The listing builds one solid part. Answer for the finished solid, in the listing's coordinates (mm). A direction names the side the tool comes from. Coordinates: 2 decimals unless noted, no trailing zeros. Write each loop counter-clockwise with the first axis right and the second up, starting at its lowest first coordinate (ties: lowest second). Pieces come first, ordered by that corner, then holes.
(1) For a pull along Z with two mould halves and no side action, classify faces 1 (the cylindrical face through (20.147, 0.986, -61.81)), 2 (the flat face through (-15.21, 0.99, 15.74)), 3 (the cylindrical face through (26.89, 0.99, 52.55)) as +Z half, -Z half, draft (parallel to the pull), parting line (faces both ways), or undercut.
(2) The part is cut by section B-B on y = 1.35. Give the number of separate pieces and of enclosed holes in the cut face, plus the area to 3 significant figures.
(3) Straight lines are drawn through the part: line 1 (X direction, y = 0.9, z = -4.5); line 2 (Z direction, x = 11, y = 0.45) (3 decimals); line 3 (Z direction, x = 3.5, y = 1.3). For each, find the intervals that lie inside material, in ascending order.
(4) The part is cut by section C-C on z = -32. Determine the outline of the cut face in (x, y), plus the area to 3 significant figures.
(5) The part is cut by section A-A on z = 9. Determine the outline of the cut face in (x, y).
(6) Which of the six approach directions +Z, -Z, +X, -X, +Y, -Y give full straight-line access (tool end or side, diameter ignored) to faces 4 (the cylindrical face through (-13.676, 0.986, 38.995)), 5 (the flat face through (35.57, 0.99, -25.22))?
(7) Given P1, Ø4, axis at x = -7.79, z = -4.5, coming from the -Y side, flat-ended and moving along its own axis, determine where the tip first touches the part or whether it passes through.
from build123d import *

# Parameters (mm, degrees)
SKETCH_1_R          = 1.65
SKETCH_1_R_2        = 5.5
EXTRUDE_1_DEPTH     = 2
SKETCH_2_R          = 1.65
CUT_EXTRUDE_1_DEPTH = 86.784644099
FILLET_1_R          = 2


with BuildPart() as part:
    # Эскиз1 → Бобышка-Вытянуть1 (new body)
    with BuildSketch(Plane(origin=(0, 0, 0), x_dir=(1, 0, 0), z_dir=(0, 1, 0))):
        with BuildLine():
            Line((22.63058135, 57.022094922), (48.869113703, -7.475462073))
            ThreePointArc((48.869113703, -7.475462073), (51.017863934, -22.940417651), (45.538728547, -37.5609872))
            ThreePointArc((45.538728547, -37.5609872), (26.585605536, -52.704925153), (3.142096023, -58.946847156))
            ThreePointArc((3.142096023, -58.946847156), (-19.13330087, -49.051718647), (-20.218209383, -24.701567755))
            Line((-20.218209383, -24.701567755), (-10.065450366, -6.533506633))
            ThreePointArc((-10.065450366, -6.533506633), (-6.891228037, 9.824000007), (9.569842381, 7.24003569))
            ThreePointArc((9.569842381, 7.24003569), (16.257964509, 34.227304723), (6.907279065, 60.411428714))
            ThreePointArc((6.907279065, 60.411428714), (9.487905153, 68.030832797), (17.329317504, 66.234391334))
            ThreePointArc((17.329317504, 66.234391334), (20.184340604, 61.745861093), (22.63058135, 57.022094922))
        make_face()
        with Locations(Location((9.550649772, -54.164426416, 0), (0, 0, 270))):
            Circle(SKETCH_1_R, mode=Mode.SUBTRACT)
        with Locations(Location((31.546703999, -45.053362436, 0), (0, 0, 90))):
            Circle(SKETCH_1_R, mode=Mode.SUBTRACT)
        with Locations(Location((0, 0, 0), (0, 0, 270))):
            Circle(SKETCH_1_R_2, mode=Mode.SUBTRACT)
        with Locations(Location((0, -9, 0), (0, 0, 270))):
            Circle(SKETCH_1_R, mode=Mode.SUBTRACT)
        with Locations(Location((-7.794228634, 4.5, 0), (0, 0, 270))):
            Circle(SKETCH_1_R, mode=Mode.SUBTRACT)
        with Locations(Location((7.794228634, 4.5, 0), (0, 0, 270))):
            Circle(SKETCH_1_R, mode=Mode.SUBTRACT)
        with BuildLine():
            Line((-5.357568053, -23.065686545), (20.09827607, -12.521530668))
            ThreePointArc((20.09827607, -12.521530668), (37.096418695, -17.67786086), (35.355339059, -35.355339059))
            ThreePointArc((35.355339059, -35.355339059), (19.134171618, -46.193976626), (0, -50))
            ThreePointArc((0, -50), (-13.730993926, -38.731264508), (-5.357568053, -23.065686545))
        make_face(mode=Mode.SUBTRACT)
    extrude(amount=EXTRUDE_1_DEPTH)

    # Эскиз2 → Вырез-Вытянуть1 (cut, through all)
    with BuildSketch(Plane.XZ):
        with Locations(Location((21.974708544, -27.113395045, 0), (0, 0, 270))):
            Circle(SKETCH_2_R)
        with Locations(Location((12.414405238, -62.792932716, 0), (0, 0, 270))):
            Circle(SKETCH_2_R)
        with Locations(Location((20.340189466, -45.796033589, 0), (0, 0, 270))):
            Circle(SKETCH_2_R)
    extrude(amount=-CUT_EXTRUDE_1_DEPTH, mode=Mode.SUBTRACT)

    # Скругление1
    fillet_1_edges = [part.edges().sort_by_distance(p)[0] for p in [
        (9.569842381, 1, -7.24003569),
    ]]
    fillet(fillet_1_edges, radius=FILLET_1_R)


solid = part.part
Model answer:
1. face 1: -Z half
1. face 2: undercut
1. face 3: +Z half
2. separate pieces: 1
2. enclosed holes: 10
2. area: 3,480 mm2
3. line 1: x = -11.12 to -9.44, -6.14 to -3.16, 3.16 to 6.14, 9.44 to 44
3. line 2: z = -68.624 to -63.643, -61.943 to -53.814, -9.826 to 16.29, 48.775 to 53.376, 54.953 to 57.997
3. line 3: z = -11.48 to -4.24, 4.24 to 19.4, 49.88 to 58.93
4. outline: (16.32, 0) - (32.81, 0) - (32.81, 2) - (16.32, 2) - close
4. area: 33.0 mm2
5. outline: (-11.44, 0) - (-1.65, 0) - (-1.65, 2) - (-11.44, 2) - close; (1.65, 0) - (49.44, 0) - (49.44, 2) - (1.65, 2) - close
6. face 4: +Y, -Y
6. face 5: -Z, +X, +Y, -Y
7. P1: stops at y = 0
